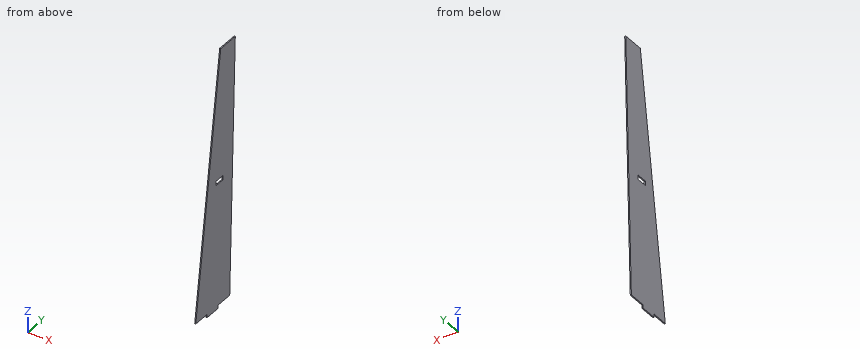
from build123d import *

# Parameters (mm, degrees)
BOSS_EXTRUDE1_DEPTH = 1.5875
CUT_EXTRUDE2_DEPTH  = 383.274521188
SKETCH4_W           = 6.35
SKETCH4_H           = 16.002
CUT_EXTRUDE3_DEPTH  = 1.5875


with BuildPart() as part:
    # Sketch1 → Boss-Extrude1 (new body)
    with BuildSketch(Plane(origin=(0, 0, 0), x_dir=(0, 0, -1), z_dir=(1, 0, 0))):
        Polygon((0, 0), (0, 31.75), (378.259807404, 19.441884667), (378.259807404, -55.234115333), align=None)
    extrude(amount=BOSS_EXTRUDE1_DEPTH)

    # Sketch3 → Cut-Extrude2 (cut, through all)
    with BuildSketch(Plane(origin=(1.5875, 0, 0), x_dir=(0, 0, -1), z_dir=(1, 0, 0))):
        Polygon((378.259807404, -55.234115333), (378.259807404, -29.834115333), (373.497307404, -29.834115333), (373.497307404, -54.538687299), align=None)
        Polygon((378.259807404, 19.441884667), (373.497307404, 19.59685064), (373.497307404, -5.958115333), (378.259807404, -5.958115333), align=None)
    extrude(amount=-CUT_EXTRUDE2_DEPTH, mode=Mode.SUBTRACT)

    # Sketch4 → Cut-Extrude3 (cut)
    with BuildSketch(Plane(origin=(1.5875, 0, 0), x_dir=(0, 0, -1), z_dir=(1, 0, 0))):
        with Locations((192.204807404, -2.939176237)):
            Rectangle(SKETCH4_W, SKETCH4_H)
    extrude(amount=-CUT_EXTRUDE3_DEPTH, mode=Mode.SUBTRACT)


solid = part.part
Work out the finished part from the listing and answer in its coordinate system (mm). Round coordinates to 2 decimals unless told otherwise and drop trailing zeros. Write each loop counter-clockwise with the first axis right and the second up, starting at its lowest first coordinate (ties: lowest second). Pieces come first, ordered by that corner, then holes. Notation, with made-up numbers: M -36.75,72 L 16.25,72 A27 ccw 16.25,94 Z; hole C -2.75,-3 d9. An arc over 180 degrees is marked long. Use a Markdown table: item, result.
1) The part is cut by section B-B on z = -220. Give the vertices of the cut face in (x, y), plus the area to 3 significant figures.
Taken from the geometry:
| item | result |
|---|---|
| outline | M 0,-32.12 L 1.59,-32.12 L 1.59,24.59 L 0,24.59 Z |
| area | 90.0 mm2 |
2) Consider line 1 (Z direction, x = 0.55, y = 0.5); line 2 (Z direction, x = 1.35, y = 12.5); line 3 (Y direction, x = 0.2, z = -203). Determine where each line is inside the solid, lowest interval first. Write a range as [from, to].
Taken from the geometry:
| item | result |
|---|---|
| line 1 | z = [-373.5, -195.38], [-189.03, 0] |
| line 2 | z = [-373.5, 0] |
| line 3 | y = [-29.64, 25.14] |
3) Flat-ended cylindrical pins translate along their axes: pin 1 (0.8 mm diameter, centred on x = 1, z = -375, fed in from -Y); pin 2 (0.5 mm diameter, centred on x = 0.5, z = -375.5, fed in from +Y). Find the tip coordinate at first contact, or state that the pin passes through.
Taken from the geometry:
| item | result |
|---|---|
| pin 1 | stops at y = -29.83 |
| pin 2 | stops at y = -5.96 |
4) The part is cut by section C-C on y = -44. Give the vertices of the cut face in (x, z).
Taken from the geometry:
| item | result |
|---|---|
| outline | M 0,-373.5 L 1.59,-373.5 L 1.59,-301.33 L 0,-301.33 Z |
5) The part is cut by section A-A on x = 1. Give the vertices of the cut face in (y, z), plus the area to 3 significant figures.
Taken from the geometry:
| item | result |
|---|---|
| outline | M -54.54,-373.5 L -29.83,-373.5 L -29.83,-378.26 L -5.96,-378.26 L -5.96,-373.5 L 19.6,-373.5 L 31.75,0 L 0,0 Z; hole M -10.94,-195.38 L 5.06,-195.38 L 5.06,-189.03 L -10.94,-189.03 Z |
| area | 19,800 mm2 |
